For this review, use the dimensioned drawing (mm, ordinates from the lowest corner) and the shaded views. Round coordinates to 2 decimals unless told otherwise and drop trailing zeros. Order: outer loops, then holes, each group sorted by start corner. A loop starts at its lowest first (then second) coordinate and runs counter-clockwise, first axis right, second up. Notation, with made-up numbers: (33, 37) - (65, 37) arc R9 cw to (65, 45) - close; hole circle Ø4 at (36.25, -9.75). An arc over 180 degrees is marked (long way). Write item = value, one per line.
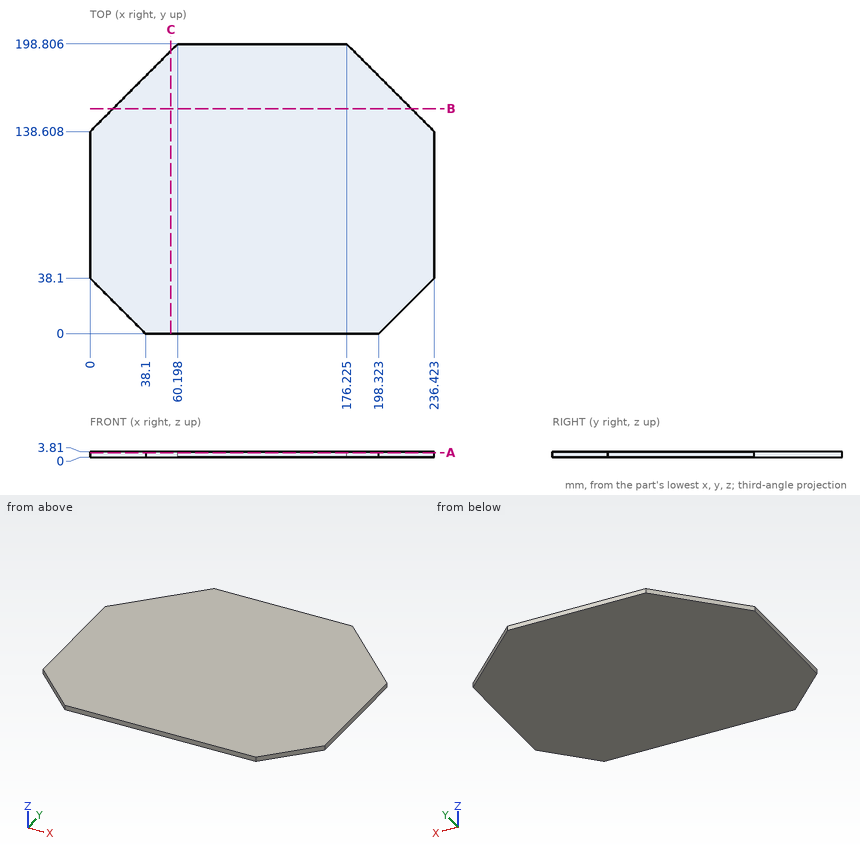
Item 1: For line 1 along Y through (x, z) = (222.5, 1); line 2 along Y through (x, z) = (42, 0.4); line 3 along X through (y, z) = (185, 2.25), list the stretches that pass through material, from the lowest coordinate up. Write a range as [from, to].
Data:
line_1 = [24.18, 152.53]
line_2 = [0, 180.61]
line_3 = [46.39, 190.03]
Item 2: Take a section at C-C, the plane x = 55.5. State the section outline as (y, z) points.
Data:
outline = (0, 0) - (194.11, 0) - (194.11, 3.81) - (0, 3.81) - close
Item 3: Take a section at A-A, the plane z = 3.05. State the section outline as (x, y) points (1 decimal).
Data:
outline = (0, 38.1) - (38.1, 0) - (198.3, 0) - (236.4, 38.1) - (236.4, 138.6) - (176.2, 198.8) - (60.2, 198.8) - (0, 138.6) - close
Item 4: Take a section at B-B, the plane y = 154.5. State the section outline as (x, z) points, and give its area (3 significant figures).
Data:
outline = (15.89, 0) - (220.53, 0) - (220.53, 3.81) - (15.89, 3.81) - close
area = 780 mm2
